from build123d import *

# Parameters (mm, degrees)
SKETCH1_W           = 5.75
SKETCH1_H           = 5.75
BOSS_EXTRUDE1_DEPTH = 2.875
CUT_EXTRUDE1_REACH  = 9.042
SKETCH2_R           = 1
SKETCH3_R           = 1.5
CUT_EXTRUDE2_DEPTH  = 8.042283011


with BuildPart() as part:
    # Sketch1 → Boss-Extrude1 (new, symmetric)
    with BuildSketch(Plane(origin=(0, 0, 0), x_dir=(1, 0, 0), z_dir=(0, 1, 0))):
        Rectangle(SKETCH1_W, SKETCH1_H)
    extrude(amount=BOSS_EXTRUDE1_DEPTH, both=True)

    # Sketch2 → Cut-Extrude1 (cut, up to next)
    with BuildSketch(Plane.XY.offset(2.875), mode=Mode.PRIVATE) as cut_extrude1_sk1:
        Circle(SKETCH2_R)
    cut_extrude1_tool1 = extrude(cut_extrude1_sk1.sketch, amount=-CUT_EXTRUDE1_REACH, mode=Mode.PRIVATE) & part.part
    add(cut_extrude1_tool1.solids().sort_by_distance((0, 0, 2.875))[0], mode=Mode.SUBTRACT)

    # Sketch3 → Cut-Extrude2 (cut, through all)
    with BuildSketch(Plane.ZY.offset(2.875)):
        Circle(SKETCH3_R)
    extrude(amount=-CUT_EXTRUDE2_DEPTH, mode=Mode.SUBTRACT)

    # Sketch4 → Cut-Revolve1 (revolve, cut)
    with BuildSketch(Plane.XY, mode=Mode.PRIVATE) as cut_revolve1_sk:
        with BuildLine():
            Line((2.625, 2.875), (5.625, 2.875))
            Line((5.625, 2.875), (5.625, -0.125))
            ThreePointArc((5.625, -0.125), (4.746320344, 1.996320344), (2.625, 2.875))
        make_face()
    cut_revolve1 = revolve(cut_revolve1_sk.sketch.rotate(Axis((0, 0, 0), (0, 1, 0)), 90), axis=Axis((0, 0, 0), (0, 1, 0)), mode=Mode.SUBTRACT)

    # Mirror1: Cut-Revolve1 across plane
    add(cut_revolve1.mirror(Plane.ZX), mode=Mode.SUBTRACT)


solid = part.part
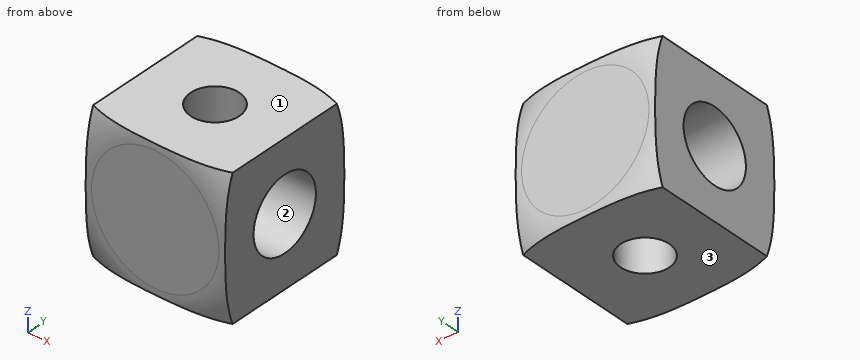
Work out the finished part from the listing and answer in its coordinate system (mm). Face numbers are marked on the shaded views. Give positions to 0.01 mm unless a question says otherwise; leave off trailing zeros. Loops run counter-clockwise (first coordinate to the right, second up) from the corner with the lowest first, then second, coordinate; pieces in that order, holes last. Notation, with made-up numbers: (45, 72) -> (52, 72) arc R27 ccw to (52, 102) -> close; hole circle Ø1 at (29.5, -40). An arc over 180 degrees is marked (long way). Use a Markdown table: item, result. Add a question column.
1) This flat-tipped pin is pushed along its axis until it touches: P1, Ø2.5, axis at x = 0, y = 0, coming from the +Z side (3 decimals). Where does it stop, or does it pass through?
2) Consider line 1 along X through (y, z) = (0, -1.8) (3 decimals); line 2 along Y through (x, z) = (0.8, 0) (3 decimals). Determine where each line is inside the solid, lowest interval first.
3) The part is cut by section A-A, the plane y = 0. Determine the outline of the cut face in (x, z) (3 decimals), plus the area to 3 significant figures.
4) For a pull along Z with two mould halves and no side action, classify the marked faces 1, 2 and 3 as +Z half, -Z half, draft (parallel to the pull), parting line (faces both ways), or undercut.
5) The part is cut by section B-B, the plane y = 1.4. Determine the outline of the cut face in (x, z) (3 decimals), plus the area to 3 significant figures.
Reported:
| question | item | result |
|---|---|---|
| 1 | P1 | stops at z = 2.875 |
| 2 | line 1 | x = -2.875 to -1, 1 to 2.875 |
| 2 | line 2 | y = -2.875 to -1.5, 1.5 to 2.875 |
| 3 | outline | (-2.875, -2.875) -> (-1, -2.875) -> (-1, -1.5) -> (-2.875, -1.5) -> close; (-2.875, 1.5) -> (-1, 1.5) -> (-1, 2.875) -> (-2.875, 2.875) -> close; (1, -2.875) -> (2.875, -2.875) -> (2.875, -1.5) -> (1, -1.5) -> close; (1, 1.5) -> (2.875, 1.5) -> (2.875, 2.875) -> (1, 2.875) -> close |
| 3 | area | 10.3 mm^2 |
| 4 | face 1 | +Z half |
| 4 | face 2 | undercut |
| 4 | face 3 | -Z half |
| 5 | outline | (-2.875, -2.875) -> (2.875, -2.875) -> (2.875, -0.539) -> (-2.875, -0.539) -> close; (-2.875, 0.539) -> (2.875, 0.539) -> (2.875, 2.875) -> (-2.875, 2.875) -> close |
| 5 | area | 26.9 mm^2 |
